Source: three-view drawing plus pictorial views. Frame: mm from the lowest corner of the part. A direction names the side the tool comes from. Round coordinates to 2 decimals unless told otherwise and drop trailing zeros. Order: outer loops, then holes, each group sorted by start corner. A loop starts at its lowest first (then second) coordinate and runs counter-clockwise, first axis right, second up. Notation, with made-up numbers: (20, 11.5) - (73, 11.5) arc R21 cw to (73, 39.5) - close; hole circle Ø1 at (49.5, 80). An arc over 180 degrees is marked (long way). Use one line per item in the form item = value. Start each with the question number.
Q1. Cut plane B-B, the plane z = 7.5. Return the cut outline in (x, y), and give its area (3 significant figures).
Q2. Draft query along Y for the marked faces 1, 2, 3 and 4. Return one class per face: released by +Y, released by -Y, zero draft, split by the parting line, or undercut.
Q3. Pin query (flat end, axial travel): pin 1 Ø5 at (x, y) = (4, 10) entering from -Z; pin 2 Ø4.5 at (y, z) = (13.5, 7.5) entering from -X; pin 3 Ø3.5 at (y, z) = (10, 7.5) entering from -X. Return the tip coordinate at first contact, or that it passes through.
Q4. Cut plane D-D, the plane y = 7.25. Return the cut outline in (x, z), and give its area (3 significant figures).
Q5. Cut plane A-A, the plane y = 10. Return the cut outline in (x, z), and give its area (3 significant figures).
Q6. Ray query, line 1 (Y direction, x = 14.6, z = 7.5); line 2 (Y direction, x = 4, z = 19.15); line 3 (X direction, y = 4.25, z = 12.5). Return the intervals inside material, ascending. Write a range as [from, to].
Q7. Set-up query: the marked faces 5 and 6. Return all of +Z, -Z, +X, -X, +Y, -Y with unobstructed straight access to the full face (end or side cutting, diameter ignored); none if empty.
Q8. Cut plane C-C, the plane x = 4. Return the cut outline in (y, z), and give its area (3 significant figures).
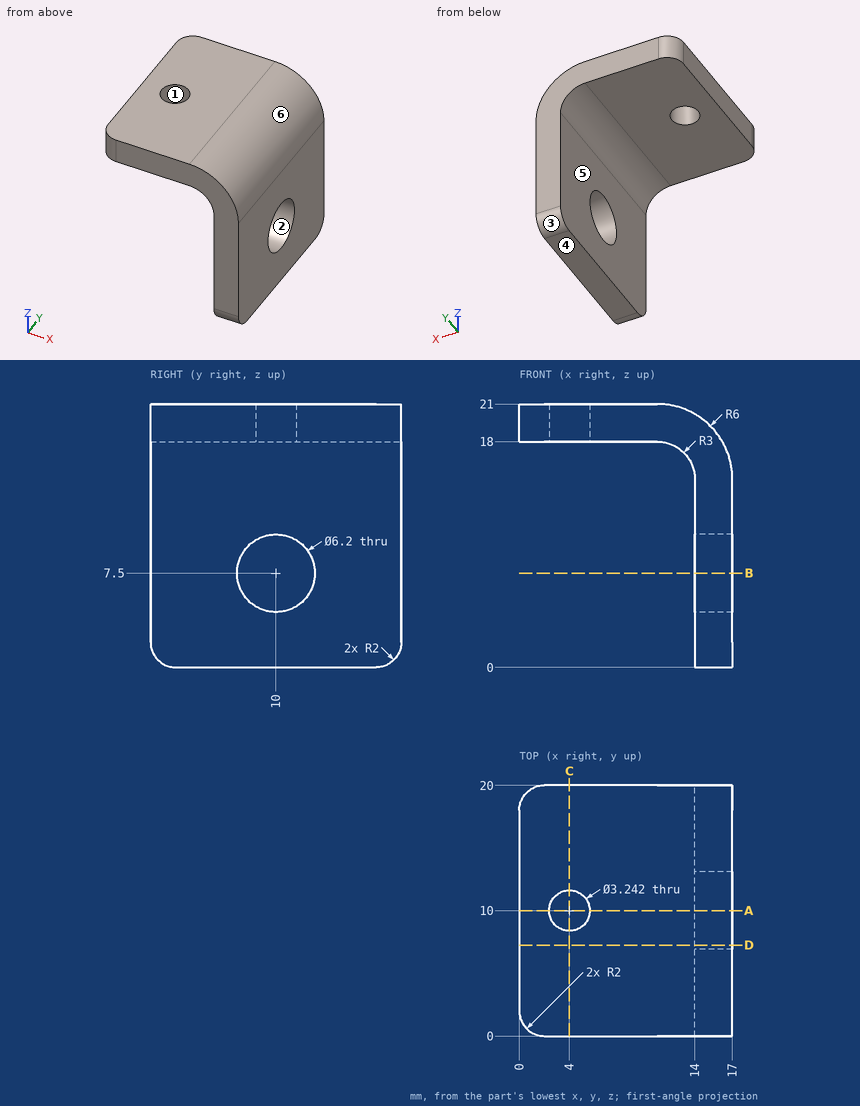
Completed:
q1.outline = (14, 0) - (17, 0) - (17, 6.9) - (14, 6.9) - close; (14, 13.1) - (17, 13.1) - (17, 20) - (14, 20) - close
q1.area = 41.4 mm2
q2.face_1 = undercut
q2.face_2 = undercut
q2.face_3 = released by +Y
q2.face_4 = zero draft
q3.pin_1 = 18
q3.pin_2 = 14
q3.pin_3 = through
q4.outline = (0, 18) - (11, 18) arc R3 cw to (14, 15) - (14, 8.93) - (17, 8.93) - (17, 15) arc R6 ccw to (11, 21) - (0, 21) - close; (14, 0) - (17, 0) - (17, 6.07) - (14, 6.07) - close
q4.area = 90.6 mm2
q5.outline = (0, 18) - (2.38, 18) - (2.38, 21) - (0, 21) - close; (5.62, 18) - (11, 18) arc R3 cw to (14, 15) - (14, 10.6) - (17, 10.6) - (17, 15) arc R6 ccw to (11, 21) - (5.62, 21) - close; (14, 0) - (17, 0) - (17, 4.4) - (14, 4.4) - close
q5.area = 70.9 mm2
q6.line_1 = [0, 6.9], [13.1, 20]
q6.line_2 = [0, 8.38], [11.62, 20]
q6.line_3 = [14, 17]
q7.face_5 = -Z, -X, +Y, -Y
q7.face_6 = +Z, +X, +Y, -Y
q8.outline = (0, 18) - (8.38, 18) - (8.38, 21) - (0, 21) - close; (11.62, 18) - (20, 18) - (20, 21) - (11.62, 21) - close
q8.area = 50.3 mm2
